Read the model definition and answer for the solid it produces. Units are mm, in the model's axes. A direction names the side the tool comes from. Round coordinates to 2 decimals unless told otherwise and drop trailing zeros. Order: outer loops, then holes, each group sorted by start corner. A loop starts at its lowest first (then second) coordinate and runs counter-clockwise, first axis right, second up. Notation, with made-up numbers: (-17.5, 6) - (-11.5, 6) arc R27 cw to (-11.5, 36) - close; hole circle Ø3 at (21, 50.5). An arc over 180 degrees is marked (long way). Put each result on its own line as item: value. Start each with the question number.
Q1. Which of the six approach directions +Z, -Z, +X, -X, +Y, -Y give full straight-line access (tool end or side, diameter ignored) to faces 4 (the face through (-12.22, 6.68, 14.55)), 5 (the face through (3.994, 1.604, -4.064))?
Q2. Section A-A on x = 0 is taken. Give the vertices of the cut face in (y, z).
Q3. Find the intervals of material crossed by line 1 along Z through (x, y) = (0, 1.25); line 2 along X through (y, z) = (5.5, 0); line 3 along Z through (x, y) = (0, 8.5), in increasing order. Write a range as from..to.
Q4. Section C-C on z = 13 is taken. Give the vertices of the cut face in (x, y).
Q5. Section B-B on z = 0 is taken. Give the vertices of the cut face in (x, y), then the cut area to 3 significant figures.
Q6. Section D-D on y = 7.25 is taken. Give the vertices of the cut face in (x, z).
Q7. For a pull along Z with two mould halves and no side action, classify faces 1 (the face through (-1.051, 6, -20)), 2 (the face through (4.206, 0.493, -4.279)), 3 (the face through (-4, 2, 4)) as pulls with the +Z half, pulls with the -Z half, needs draft (parallel to the pull), parting line crosses it, or undercut.
Q8. Each of these flat-tipped pins is pushed along its axis until it touches: pin 1 Ø2 at (x, y) = (-14, 5.5) entering from +Z; pin 2 Ø6 at (x, z) = (0, 0) entering from +Y; pin 3 Ø1.5 at (x, y) = (7, 6.5) entering from +Z; pin 4 Ø1 at (x, y) = (4, 3) entering from +Z. Where does it stop, or does it pass through?
Autodesk Inventor part; units mm, degrees
ref_plane "YZ Plane" through (0, 0, 0) normal (1, 0, 0) x (0, 1, 0)
ref_plane "XZ Plane" through (0, 0, 0) normal (0, 1, 0) x (-1, 0, 0)
ref_plane "XY Plane" through (0, 0, 0) normal (0, 0, 1) x (1, 0, 0)
sketch "Sketch9" plane through (0, 0, 0) normal (0, 1, 0) x (-1, 0, 0)
  line L0 (21, 0) -> (-21, 0) construction
  line L1 (0, 21) -> (0, -21) construction
  line L2 (21, -1) -> (20.9762, -1)
  line L3 (21, 1) -> (20.9762, 1)
  line L4 (-20.9762, 1) -> (-21, 1)
  line L5 (1, 21) -> (1, 20.9762)
  line L6 (1, -20.9762) -> (1, -21)
  line L7 (-1, 21) -> (-1, 20.9762)
  line L8 (-1, -5.9161) -> (-1, -21)
  line L9 (-5.9161, -1) -> (-18.9762, -1)
  circle A0 centre (0, 0) radius 5
  arc A1 (-5.9161, -1) -> (-1, -5.9161) centre (0, 0) ccw
  line L10 (-20.9762, -1) -> (-18.9762, -1)
  line L11 (1, -21) -> (1, -3.873) construction
  line L12 (-3.873, 1) -> (-18.9762, 1) construction
  line L13 (-18.9762, 1) -> (-20.9762, 1) construction
  line L14 (-3.873, 1) -> (20.9762, 1) construction
  line L15 (-5.9161, -1) -> (20.9762, -1) construction
  line L16 (1, -3.873) -> (1, 20.9762) construction
  line L17 (-1, -5.9161) -> (-1, 20.9762) construction
  line L18 (0, 21) -> (0, 19) construction
  line L19 (0, 19) -> (1, 19) construction
  arc A2 (-1, -20.9762) -> (0, 21) centre (0, 0) ccw construction
  arc A3 (20.9762, 1) -> (-20.9762, -1) centre (0, 0) ccw construction
  arc A4 (-1, -18.9737) -> (-18.9737, -1) centre (0, 0) ccw
  line L20 (-1, 19) -> (1, 19)
  point P0 (-4.899, -1)
  point P1 (-1, -4.899)
  dimension "d35" = 10
  dimension "d50" = 2
  dimension "d53" = 38
extrude "Extrusion5" add sketch "Sketch9" along normal blind 2
chamfer "Chamfer1" distance 0.5 distance2 1 1 edges at (4.2426, 2, -4.2426) measured on face at (13.5988, 2, 4.219)
sketch "Sketch12" plane through (0, 0, 0) normal (0, 1, 0) x (-1, 0, 0)
  arc A0 (1.0513, -20.9737) -> (-20.9762, -1) centre (0, 0) ccw
  circle A1 centre (0, 0) radius 5
  arc A2 (1, -18.9737) -> (-18.9737, -1) centre (0, 0) ccw
  line L0 (-18.9737, -1) -> (-5.4083, -1)
  line L1 (-18.9737, -1) -> (-20.9762, -1)
  line L2 (-1, -5.4083) -> (-1, -18.9737)
  line L3 (0.0513, 20.9999) -> (0.0513, -20.9999) construction
  line L4 (1.0513, 21.0025) -> (1.0513, -20.9975) construction
  line L5 (1.0513, -20.9737) -> (1.0513, -18.9737)
  arc A3 (-1, -18.9737) -> (-18.9737, -1) centre (0, 0) ccw
  line L6 (1.0513, -18.9737) -> (-1, -18.9737)
  line L7 (1.0513, -18.9737) -> (1.0513, -18.9709)
  dimension "d58" = 42
  dimension "d60" = 19
  dimension "d63" = 1
  dimension "d64" = 2
extrude "Extrusion8" add sketch "Sketch12" along normal blind 11.5 contours L5 L7 A2 L1 A0
properties part number "base layer 4"
Findings:
1. face 4: +Y
1. face 5: -Z, +X, +Y
2. outline: (0, -19) - (2, -19) - (2, -5) - (0, -5) - close; (0, 5) - (2, 5) - (2, 19) - (11.5, 19) - (11.5, 21) - (0, 21) - close
3. line 1: -19..-5, 5..21
3. line 2: -21..-19, 19..21
3. line 3: 19..21
4. outline: (-16.49, 0) - (16.49, 0) - (16.49, 11.5) - (13.86, 11.5) - (13.86, 2) - (-13.86, 2) - (-13.86, 11.5) - (-16.49, 11.5) - close
5. outline: (-21, 0) - (-5, 0) - (-5, 2) - (-19, 2) - (-19, 11.5) - (-21, 11.5) - close; (5, 0) - (21, 0) - (21, 11.5) - (19, 11.5) - (19, 2) - (5, 2) - close
5. area: 102 mm2
6. outline: (-1.05, -20.97) - (-1.05, -18.97) arc R19 cw (long way) to (18.97, -1) - (20.98, -1) arc R21 ccw (long way) to start
7. face 1: needs draft
7. face 2: pulls with the -Z half
7. face 3: undercut
8. pin 1: z = 16.49
8. pin 2: through
8. pin 3: z = 20.05
8. pin 4: z = 20.71
